Verification items for the finished model (mm, model axes). A direction names the side the tool comes from. Give positions to 0.01 mm unless a question says otherwise; leave off trailing zeros. Order: outer loops, then holes, each group sorted by start corner. A loop starts at its lowest first (then second) coordinate and runs counter-clockwise, first axis right, second up. Notation, with made-up numbers: M 2.25,-25 L 8.25,-25 A32 ccw 8.25,11 Z; hole C -35.5,38.5 d11. An arc over 180 degrees is marked long. Answer as a JSON object with one key per item and string values.
Autodesk Inventor part; units mm, degrees
ref_plane "YZ Plane" through (0, 0, 0) normal (1, 0, 0) x (0, 1, 0)
ref_plane "XZ Plane" through (0, 0, 0) normal (0, 1, 0) x (-1, 0, 0)
ref_plane "XY Plane" through (0, 0, 0) normal (0, 0, 1) x (1, 0, 0)
sketch "Sketch1" plane through (0, 0, 0) normal (0, 1, 0) x (-1, 0, 0)
  line L0 (0, 0) -> (0, 6)
  line L1 (-3, 0) -> (-3, 6)
  line L2 (-3, 6) -> (-5, 6)
  line L3 (-5, 6) -> (-5, 1.5)
  line L4 (-5, 1.5) -> (-6, 1.5)
  line L5 (-6, 1.5) -> (-6, 0)
  line L6 (-6, 0) -> (-3, 0)
  dimension "InsideDiameter" = 6
  dimension "OuterDiameter" = 10
  dimension "FlangeDiameter" = 12
  dimension "FlangeThickness" = 1.5
  dimension "Length" = 6
revolve "Revolution1" add sketch "Sketch1" angle 360 about axis through (0, 0, 0) along (0, 0, 1)
chamfer "Chamfer1" distance 0.3 angle 45 1 edges at (-3, 0, 0)
chamfer "Chamfer2" distance 0.5 angle 45 1 edges at (-3, 0, 6)
chamfer "Chamfer3" distance 0.3 distance2 1 1 edges at (-5, 0, 6) measured on face at (4.4516, -0.3989, 6)
sketch "Sketch2" plane through (0, 0, 6) normal (0, 0, 1) x (1, 0, 0)
  circle A0 centre (0, 0) radius 5
  line L0 (-2.3749, -4.4) -> (2.3749, -4.4)
  line L1 (-5, 0) -> (5, 0) construction
  line L2 (-2.3749, 4.4) -> (2.3749, 4.4)
  dimension "Width" = 8.8
extrude "Extrusion1" cut sketch "Sketch2" against normal up to surface (4.5 mm away) contours L2 A0 | A0 L0
properties part number "LED-0606" material "Acetal Resin, Black"
Q1. Material ranges on L1, parallel to Y at x = 0, z = 3.15; L2, parallel to Z at x = 5.25, y = -2.5; L3, parallel to X at y = 0.5, z = 4, recorded low to high.
Resolved:
{"L1": "y = -4.4 to -3, 3 to 4.4", "L2": "z = 0 to 1.5", "L3": "x = -4.97 to -2.96, 2.96 to 4.97"}
Q2. Section check D-D on z = 0.5. Record the cut outline in (x, y).
Resolved:
{"outline": "C 0,0 d12; hole C 0,0 d6"}
Q3. Release check for a two-part mould opening along X. For faces 5 (the face through (-5, 0, 3)), 6 (the face through (-2.2, 3, 6)), 7 (the face through (-3, 0, 3)) record: +X half, -X half, draft (parallel to the pull), parting line (faces both ways), or undercut.
Resolved:
{"face 5": "-X half", "face 6": "draft", "face 7": "undercut"}
Q4. Section check B-B on y = 0. Record the cut outline in (x, z), then the cut area to 3 significant figures.
Resolved:
{"outline": "M -6,0 L -3.3,0 L -3,0.3 L -3,5.5 L -3.5,6 L -4.7,6 L -5,5 L -5,1.5 L -6,1.5 Z; M 3,0.3 L 3.3,0 L 6,0 L 6,1.5 L 5,1.5 L 5,5 L 4.7,6 L 3.5,6 L 3,5.5 Z", "area": "26.4 mm²"}
Q5. Tool access check on faces 1 (the face through (-4.75, -0.08, 5.83)), 2 (the face through (5, 0, 3)), 3 (the face through (0, -4.4, 4)), 4 (the face through (0, 4.4, 4)). Record the directions out of +Z, -Z, +X, -X, +Y, -Y that give a thin tool (end or side, any length) a straight path to the whole face; none if there is none.
Resolved:
{"face 1": "+Z, -X", "face 2": "+Z, +X", "face 3": "+Z, +X, -X, -Y", "face 4": "+Z, +X, -X, +Y"}
Q6. Gauge pin test, flat ends, axial feed: pin 1 Ø3 at (x, z) = (-2.5, 1.5) entering from +Y; pin 2 Ø3 at (x, z) = (4, 5) entering from -Y; pin 3 Ø6 at (x, y) = (-0.5, -4) entering from -Z; pin 4 Ø1.4 at (x, z) = (1, 3) entering from -Y. Record the tip position at first contact, or that the pin passes through.
Resolved:
{"pin 1": "stops at y = 5.92", "pin 2": "stops at y = -4.33", "pin 3": "stops at z = 0", "pin 4": "stops at y = -4.4"}
Q7. Section check C-C on z = 5.25. Record the cut outline in (x, y) (3 decimals).
Resolved:
{"outline": "M -2.213,-4.4 L 2.213,-4.4 A4.925 ccw 2.213,4.4 L -2.213,4.4 A4.925 ccw Z; hole C 0,0 d6"}
Q8. Section check A-A on x = 0. Record the cut outline in (y, z).
Resolved:
{"outline": "M -6,0 L -3.3,0 L -3,0.3 L -3,5.5 L -3.5,6 L -4.4,6 L -4.4,1.5 L -6,1.5 Z; M 3,0.3 L 3.3,0 L 6,0 L 6,1.5 L 4.4,1.5 L 4.4,6 L 3.5,6 L 3,5.5 Z"}
